Input: dimensioned drawing with shaded views. Units: mm. Origin: part minimum x, y, z. A direction names the side the tool comes from. Round coordinates to 2 decimals unless told otherwise and drop trailing zeros. Order: outer loops, then holes, each group sorted by start corner. A loop starts at its lowest first (then second) coordinate and runs counter-clockwise, first axis right, second up. Notation, with made-up numbers: M 49.25,10 L 73.25,10 A12 cw 73.25,29 Z; hole C 42,-15.75 d1. An arc over 180 degrees is marked long. One line per question, with ' | ' between items.
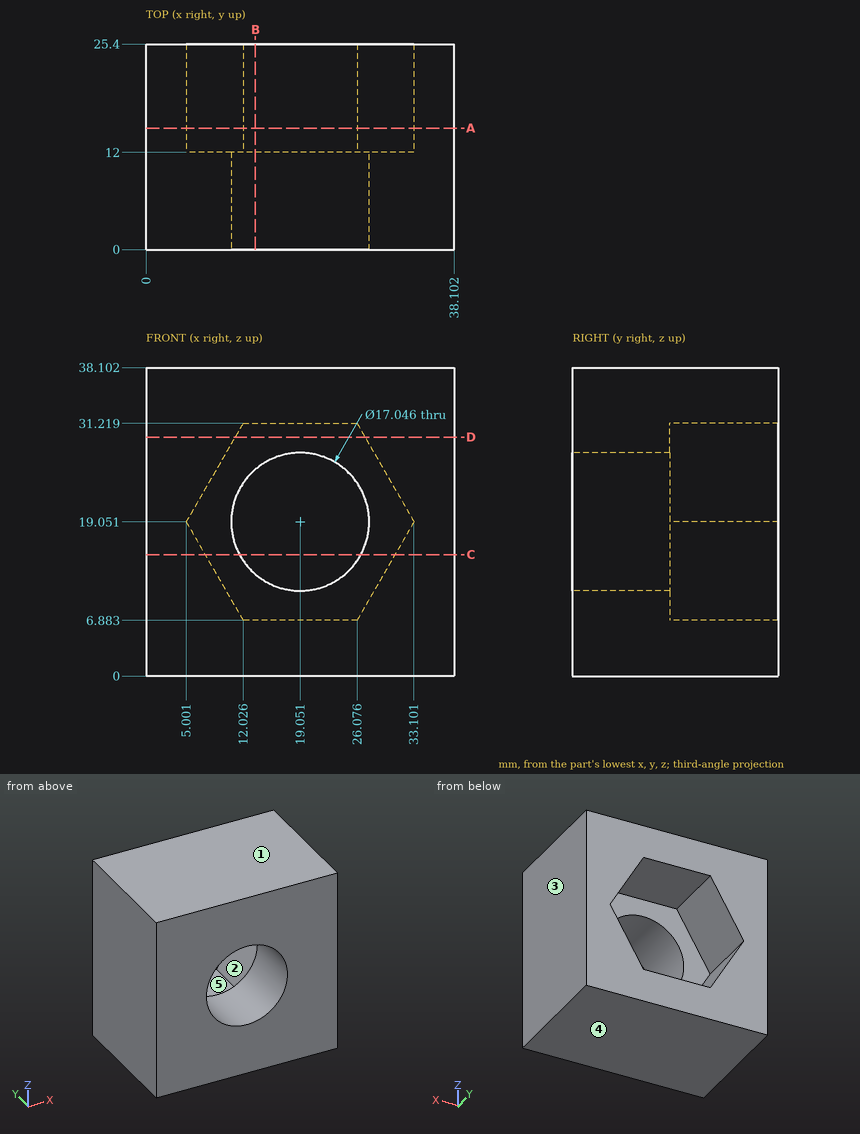
Item 1: First-contact query: pin 1 (8 mm diameter, centred on x = 12, z = 17, fed in from +Y). Flat tip, straight axial feed; report the tip coordinate or a pass-through.
Report:
pin 1: y = 12
Item 2: Line query: line 1 along X through (y, z) = (21.5, 9.5) (1 decimal); line 2 along Z through (x, y) = (22.5, 18.5); line 3 along X through (y, z) = (17.5, 16.5) (1 decimal). Output: solid intervals per line, ascending. Write a range as from..to.
Report:
line 1: 0..10.5, 27.6..38.1 | line 2: 0..6.88, 31.22..38.1 | line 3: 0..6.5, 31.6..38.1
Item 3: Access query for the marked faces 4 and 5. Directions: +Z, -Z, +X, -X, +Y, -Y. A direction counts if a zero-diameter tool reaches every point of the face in a straight line with its end or side. Return the directions, or none.
Report:
face 4: -Z, +X, -X, +Y, -Y | face 5: +Y
Item 4: Section query A-A, the plane y = 15. Return loops of the section in (x, z).
Report:
outline: M 0,0 L 38.1,0 L 38.1,38.1 L 0,38.1 Z; hole M 5,19.05 L 12.03,6.88 L 26.08,6.88 L 33.1,19.05 L 26.08,31.22 L 12.03,31.22 Z
Item 5: Section query B-B, the plane x = 13.5. Return loops of the section in (y, z).
Report:
outline: M 0,0 L 25.4,0 L 25.4,6.88 L 12,6.88 L 12,12.58 L 0,12.58 Z; M 0,25.52 L 12,25.52 L 12,31.22 L 25.4,31.22 L 25.4,38.1 L 0,38.1 Z
Item 6: Mould query, pull axis X, two halves, no side actions, for the marked faces 1, 2 and 3. Classes: +X half, -X half, draft (parallel to the pull), parting line (faces both ways), or undercut.
Report:
face 1: draft | face 2: undercut | face 3: +X half
Item 7: Section query D-D, the plane z = 29.5. Return loops of the section in (x, y).
Report:
outline: M 0,0 L 38.1,0 L 38.1,25.4 L 27.07,25.4 L 27.07,12 L 11.03,12 L 11.03,25.4 L 0,25.4 Z
Item 8: Section query C-C, the plane z = 15. Return loops of the section in (x, y).
Report:
outline: M 0,0 L 11.55,0 L 11.55,12 L 7.34,12 L 7.34,25.4 L 0,25.4 Z; M 26.55,0 L 38.1,0 L 38.1,25.4 L 30.76,25.4 L 30.76,12 L 26.55,12 Z
